from build123d import *

# Parameters (mm, degrees)
F0_W     = 200
F0_H     = 200
F1_DEPTH = 5
F3_ANGLE = 180
F4_W     = 65
F4_H     = 65
F5_DEPTH = 15
F5_TAPER = 35


with BuildPart() as f1:
    # F0 (on Top) → F1 (new body)
    with BuildSketch(Plane.XY):
        Rectangle(F0_W, F0_H)
    extrude(amount=-F1_DEPTH)

    # F2 (on Top) → F3 (revolve)
    with BuildSketch(Plane.XY):
        with BuildLine():
            Line((-87.5, 50), (-12.5, 50))
            ThreePointArc((-12.5, 50), (-50, 87.5), (-87.5, 50))
        make_face()
    revolve(axis=Axis((-50, 50, 0), (1, 0, 0)), revolution_arc=F3_ANGLE)

    # F4 (on Top) → F5 (join)
    with BuildSketch(Plane.XY):
        with Locations((50, 50)):
            Rectangle(F4_W, F4_H)
    extrude(amount=F5_DEPTH, taper=F5_TAPER)

    # F7 (on plane+point) → F8 (revolve)
    with BuildSketch(Plane.XZ.offset(50)):
        with BuildLine():
            Line((-87.5, 0), (-67.5, 0))
            ThreePointArc((-67.5, 0), (-77.5, 10), (-87.5, 0))
        make_face()
    revolve(axis=Axis((-50, -50, -2.7900552377), (0, 0, -1)))

    # F9 (on plane+point) → F10 (revolve)
    with BuildSketch(Plane.XZ.offset(50)):
        Polygon((50, 37.5), (12.5, 0), (50, 0), align=None)
    revolve(axis=Axis((50, -50, 18.75), (0, 0, 1)))


solid = f1.part
Build history of the part. All positions in model axes, mm. A direction names the side the tool comes from. Round coordinates to 2 decimals unless told otherwise and drop trailing zeros. Write each loop counter-clockwise with the first axis right and the second up, starting at its lowest first coordinate (ties: lowest second). Pieces come first, ordered by that corner, then holes. Notation, with made-up numbers: (-32.5, -3.5) - (15.5, -3.5) arc R16 ccw to (15.5, 15.5) - close; hole circle Ø4 at (72, 60). An arc over 180 degrees is marked (long way). Use CSV: the item, a comma, the result in double quotes.
(1) Band-saw the part on A-A (y = 39.5). Write the cut outline in (x, z).
Response:
outline,"(-100, -5) - (100, -5) - (100, 0) - (82.5, 0) - (72, 15) - (28, 15) - (17.5, 0) - (-14, 0) arc R36 ccw to (-86, 0) - (-100, 0) - close"
(2) Wall check: line 1 (X direction, y = 45, z = 12); line 2 (Z direction, x = 55, y = -5.5); line 3 (Z direction, x = 56.5, y = 49). Give the ranges that are in metal, low to high.
Response:
line 1,"-85.17 to -14.83, 25.9 to 74.1"
line 2,"-5 to 0"
line 3,"-5 to 15"
(3) Band-saw the part on B-B (z = 26). Write the cut outline in (x, y), plus the area to 3 significant figures.
Response:
outline,"circle Ø54.05 at (-50, 50); circle Ø23 at (50, -50)"
area,"2,710 mm²"
(4) Band-saw the part on C-C (x = -10). Write the cut outline in (y, z).
Response:
outline,"(-100, -5) - (100, -5) - (100, 0) - (-100, 0) - close"
(5) 3-axis set-ups, long thin cutter, end or side, ignore diameter. For faces 4 (the flat face through (22.68, 49.54, 7.4)), 5 (the flat face through (50.46, 22.68, 7.4)), 6 (the flat face through (-50, -50, 0)), 7 (the flat face through (49.54, 77.32, 7.4)): which of +Z, -Z, +X, -X, +Y, -Y reach the whole face in a straight line?
Response:
face 4,"+Z, +Y"
face 5,"+Z, +X"
face 6,"+Z"
face 7,"+Z, +X, +Y"
(6) Pin check, flat tips, straight feed: P1, Ø1.5, axis at x = -15, y = -11.5, coming from the +Z side; P2, Ø8, axis at x = -40, z = 8, coming from the +Y side; P3, Ø10, axis at x = 50.5, z = 23, coming from the -Y side. Stop position of each tip, or through.
Response:
P1,"z = 0"
P2,"y = 86.45"
P3,"y = -69.49"
(7) Mould opens along X. For faces 1 (the flat face through (77.32, 50.46, 7.4)), 2 (the flat face through (50, 50, 15)), 3 (the flat face through (-1, 1, 0)) say: pulls with the +X half, pulls with the -X half, needs draft (parallel to the pull), parting line crosses it, or undercut.
Response:
face 1,"pulls with the +X half"
face 2,"needs draft"
face 3,"undercut"
